Input: part model. Units: mm. Frame: model coordinates. A direction names the side the tool comes from. Coordinates: 2 decimals unless noted, no trailing zeros. Write each loop counter-clockwise with the first axis right and the second up, starting at its lowest first coordinate (ties: lowest second). Pieces come first, ordered by that corner, then holes. Notation, with made-up numbers: (23, -18.75) - (47, -18.75) arc R25 cw to (47, 1.25) - close; hole circle Ø4 at (45, 48). An arc over 180 degrees is marked (long way). Use CSV: the item, a comma, the result in double quotes.
```python
from build123d import *

# Parameters (mm, degrees)
SKETCH_1_W      = 50
SKETCH_1_H      = 3
EXTRUDE_1_DEPTH = 3


with BuildPart() as part:
    # 草圖1 → 填料-伸長1 (new body)
    with BuildSketch(Plane.XY):
        with BuildLine():
            Line((-5, 40), (-15, 40))
            ThreePointArc((-15, 40), (-32.67766953, 32.67766953), (-40, 15))
            Line((-40, 15), (-40, 5))
            Line((-40, 5), (-37, 5))
            Line((-37, 5), (-37, -5))
            Line((-37, -5), (-40, -5))
            Line((-40, -5), (-40, -15))
            ThreePointArc((-40, -15), (-32.67766953, -32.67766953), (-15, -40))
            Line((-15, -40), (-5, -40))
            Line((-5, -40), (-5, -37))
            Line((-5, -37), (5, -37))
            Line((5, -37), (5, -40))
            Line((5, -40), (15, -40))
            ThreePointArc((15, -40), (32.67766953, -32.67766953), (40, -15))
            Line((40, -15), (40, -5))
            Line((40, -5), (37, -5))
            Line((37, -5), (37, 5))
            Line((37, 5), (40, 5))
            Line((40, 5), (40, 15))
            ThreePointArc((40, 15), (32.67766953, 32.67766953), (15, 40))
            Line((15, 40), (5, 40))
            Line((5, 40), (5, 37))
            Line((5, 37), (-5, 37))
            Line((-5, 37), (-5, 40))
        make_face()
        Rectangle(SKETCH_1_W, SKETCH_1_H, mode=Mode.SUBTRACT)
    extrude(amount=EXTRUDE_1_DEPTH)


solid = part.part
```
(1) Cut plane A-A on x = 16. Return loops of the section in (y, z).
Check values:
outline,"(-39.98, 0) - (-1.5, 0) - (-1.5, 3) - (-39.98, 3) - close; (1.5, 0) - (39.98, 0) - (39.98, 3) - (1.5, 3) - close"
(2) Cut plane C-C on x = -13.5. Return loops of the section in (y, z).
Check values:
outline,"(-40, 0) - (-1.5, 0) - (-1.5, 3) - (-40, 3) - close; (1.5, 0) - (40, 0) - (40, 3) - (1.5, 3) - close"
(3) Reachability of faces 5 (the flat face through (-5, 38, 1)), 6 (the flat face through (-38, -5, 1)), 7 (the flat face through (0, 1.5, 1)), 8 (the flat face through (0, -37, 1)), 9 (the flat face through (39, -5, 1)) from +Z, -Z, +X, -X, +Y, -Y: full face, straight path, thin tool, end or side. Return the list, or none.
Check values:
face 5,"+Z, -Z, +Y"
face 6,"+Z, -Z, -X"
face 7,"+Z, -Z"
face 8,"+Z, -Z, -Y"
face 9,"+Z, -Z, +X"
(4) Pin query (flat end, axial travel): pin 1 Ø1.5 at (x, z) = (0, 2.5) entering from +Y; pin 2 Ø1.5 at (y, z) = (0, 2) entering from +X; pin 3 Ø1.5 at (y, z) = (38.5, 1.5) entering from -X. Return the tip coordinate at first contact, or that it passes through.
Check values:
pin 1,"y = 37"
pin 2,"x = 37"
pin 3,"x = -25.37"
(5) Draft query along X for faces 1 (the flat face through (-40, 10, 1)), 2 (the flat face through (40, -10, 1)), 3 (the flat face through (-1, 9, 3)), 4 (the flat face through (5, -38, 1)). Return one class per face: pulls with the +X half, pulls with the -X half, needs draft (parallel to the pull), parting line crosses it, or undercut.
Check values:
face 1,"pulls with the -X half"
face 2,"pulls with the +X half"
face 3,"needs draft"
face 4,"undercut"
(6) Cut plane D-D on y = -3.5. Return loops of the section in (x, z).
Check values:
outline,"(-37, 0) - (37, 0) - (37, 3) - (-37, 3) - close"
(7) Ray query, probe 1 along Y at (x, z) = (-14, 2.3); probe 2 along Y at (x, z) = (2, 2.85); probe 3 along X at (y, z) = (15.5, 2.7) (3 decimals). Return the intervals inside material, ascending. Write a range as from..to.
Check values:
probe 1,"-40..-1.5, 1.5..40"
probe 2,"-37..-1.5, 1.5..37"
probe 3,"-39.995..39.995"
(8) Cut plane B-B on z = 1. Return loops of the section in (x, y), and give its area (3 significant figures).
Check values:
outline,"(-40, -15) arc R25 ccw to (-15, -40) - (-5, -40) - (-5, -37) - (5, -37) - (5, -40) - (15, -40) arc R25 ccw to (40, -15) - (40, -5) - (37, -5) - (37, 5) - (40, 5) - (40, 15) arc R25 ccw to (15, 40) - (5, 40) - (5, 37) - (-5, 37) - (-5, 40) - (-15, 40) arc R25 ccw to (-40, 15) - (-40, 5) - (-37, 5) - (-37, -5) - (-40, -5) - close; hole (-25, -1.5) - (25, -1.5) - (25, 1.5) - (-25, 1.5) - close"
area,"5,590 mm^2"
